Design review of the part shown in the three views and the two pictorial views. Dimensions are in mm from the part's minimum x, y and z. A direction names the side the tool comes from. Round coordinates to 2 decimals unless told otherwise and drop trailing zeros. Write each loop counter-clockwise with the first axis right and the second up, starting at its lowest first coordinate (ties: lowest second). Pieces come first, ordered by that corner, then holes. Notation, with made-up numbers: (62, -35.75) -> (115, -35.75) arc R15 ccw to (115, -21.75) -> close; hole circle Ø7 at (1, 15.5). An arc over 180 degrees is marked (long way). Answer as a JSON object with one key per item and string values. Group by question number.
1) We need section C-C, the plane y = 9. Write out the cut boundary in (x, z), then the cut area to 3 significant figures.
2) We need section D-D, the plane x = 49.5. Write out the cut boundary in (y, z).
3) We need section B-B, the plane z = 15. Write out the cut boundary in (x, y), then the cut area to 3 significant figures.
4) Mouldability with a two-part tool opening along Z and no side actions: class the marked faces 3, 4 and 5 as pulls with the +Z half, pulls with the -Z half, needs draft (parallel to the pull), parting line crosses it, or undercut.
5) We need section A-A, the plane x = 11. Write out the cut boundary in (y, z).
6) Machinability: for the marked faces 1 and 2, which of the approach directions +Z, -Z, +X, -X, +Y, -Y give a long, thin tool a straight path to every point of the face, cutting with its end or side? Answer none if there is none.
7) To check wall thickness, follow probe 1 along X at (y, z) = (1.75, 17.5); probe 2 along Z at (x, y) = (50, 22). State the ranges of each line that lie inside material, in increasing order. Write a range as [from, to].
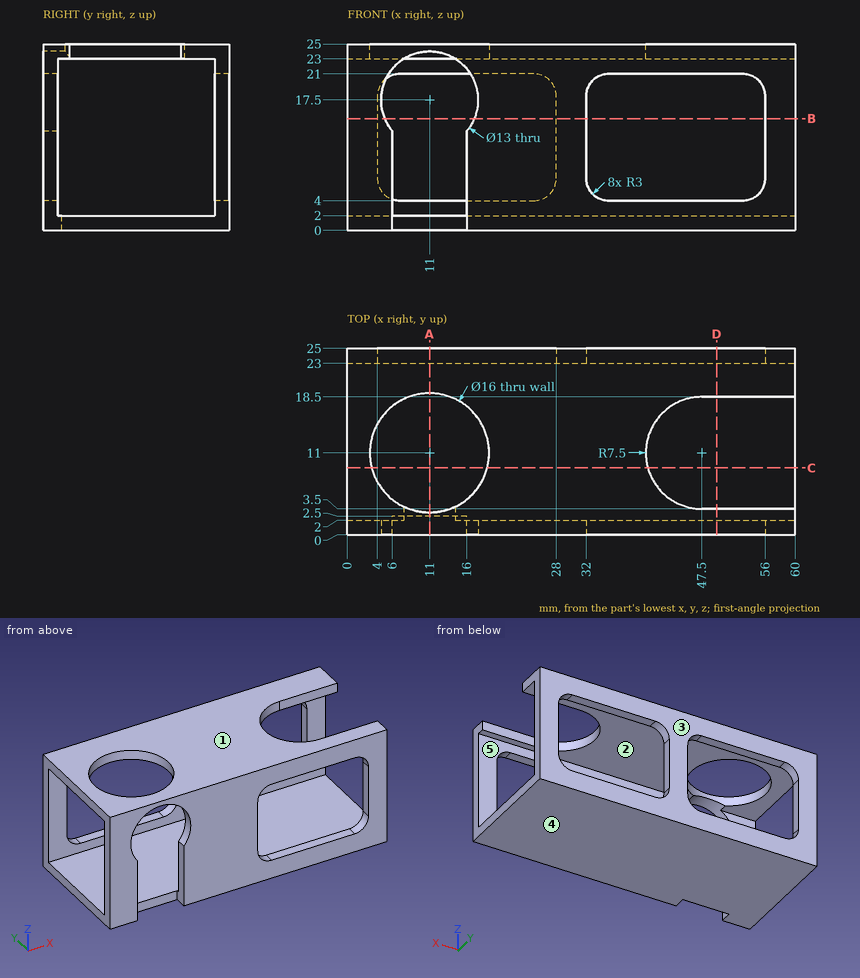
Here are the results:
{
 "1": {"outline": "(0, 0) -> (60, 0) -> (60, 2) -> (0, 2) -> close; (0, 23) -> (3.25, 23) -> (3.25, 25) -> (0, 25) -> close; (18.75, 23) -> (40.27, 23) -> (40.27, 25) -> (18.75, 25) -> close", "area": "170 mm^2"},
 "2": {"outline": "(0, 0) -> (25, 0) -> (25, 4) -> (23, 4) -> (23, 2) -> (2, 2) -> (2, 4) -> (0, 4) -> close; (0, 21) -> (2, 21) -> (2, 23) -> (3.5, 23) -> (3.5, 25) -> (0, 25) -> close; (18.5, 23) -> (23, 23) -> (23, 21) -> (25, 21) -> (25, 25) -> (18.5, 25) -> close"},
 "3": {"outline": "(0, 0) -> (5, 0) -> (5, 2) -> (0, 2) -> close; (0, 23) -> (4, 23) -> (4, 25) -> (0, 25) -> close; (17, 0) -> (32, 0) -> (32, 2) -> (17, 2) -> close; (28, 23) -> (32, 23) -> (32, 25) -> (28, 25) -> close; (56, 0) -> (60, 0) -> (60, 2) -> (56, 2) -> close; (56, 23) -> (60, 23) -> (60, 25) -> (56, 25) -> close", "area": "72.0 mm^2"},
 "4": {"face 3": "needs draft", "face 4": "pulls with the -Z half", "face 5": "undercut"},
 "5": {"outline": "(0, 24) -> (3, 24) -> (3, 25) -> (0, 25) -> close; (2.5, 0) -> (25, 0) -> (25, 4) -> (23, 4) -> (23, 2) -> (2.5, 2) -> close; (19, 23) -> (23, 23) -> (23, 21) -> (25, 21) -> (25, 25) -> (19, 25) -> close"},
 "6": {"face 1": "+Z, +X, -X, +Y, -Y", "face 2": "+X, -X"},
 "7": {"probe 1": "x = [0, 4.5], [17.5, 32], [56, 60]", "probe 2": "z = [0, 2], [23, 25]"}
}
